Geometry: see drawing. Coordinates: mm, zero at the bounding-box minimum. A direction names the side the tool comes from. Round coordinates to 2 decimals unless told otherwise and drop trailing zeros. Loops run counter-clockwise (first coordinate to the right, second up) from the corner with the lowest first, then second, coordinate; pieces in that order, holes last. Notation, with made-up numbers: M -8.5,-13.75 L 0.5,-13.75 A31 cw 0.5,23.25 Z; hole C 45.5,54.25 d8. An arc over 180 degrees is marked long. Answer as a JSON object with one key per item and string values.
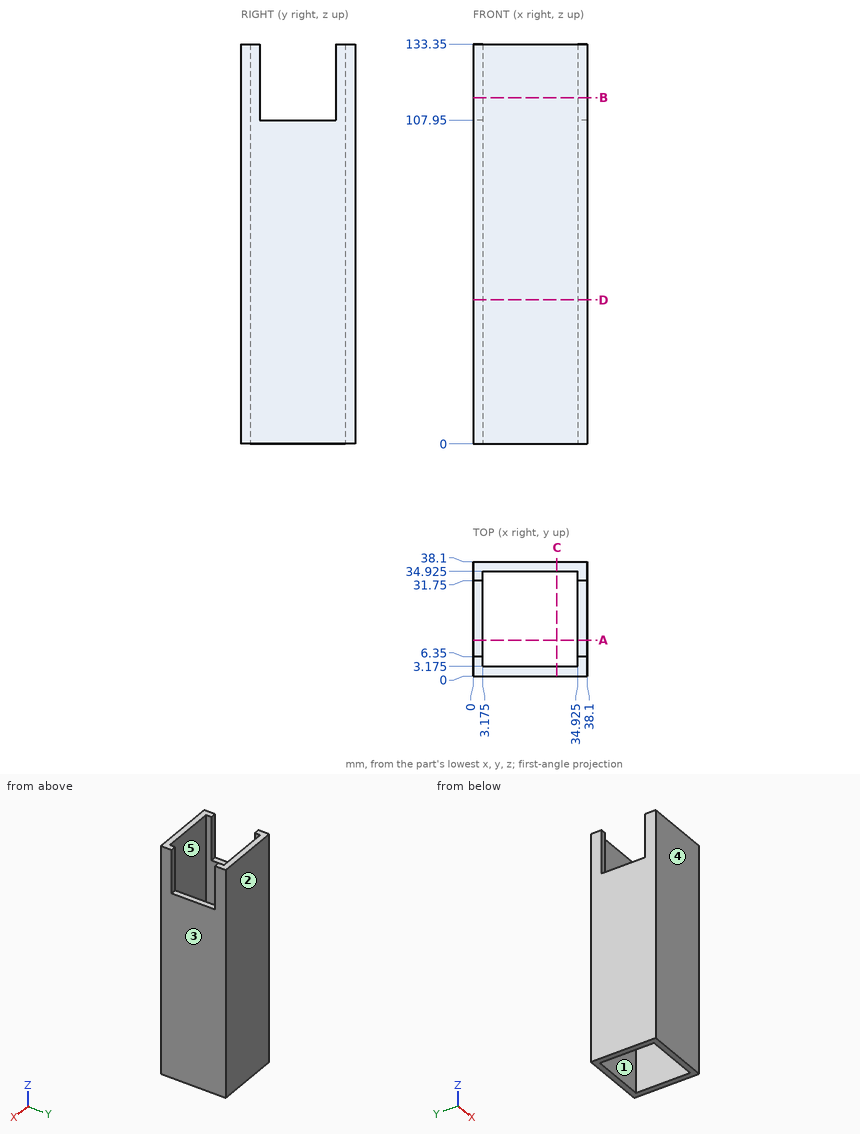
1) Pin query (flat end, axial travel): P1, Ø1.6, axis at x = 36.5, y = 14.5, coming from the +Z side. Return the tip coordinate at first contact, or that it passes through.
Results:
{"P1": "z = 107.95"}
2) Section query B-B (z = 115.5). Return the cut outline in (x, y) (3 decimals).
Results:
{"outline": "M 0,0 L 38.1,0 L 38.1,6.35 L 34.925,6.35 L 34.925,3.175 L 3.175,3.175 L 3.175,6.35 L 0,6.35 Z; M 0,31.75 L 3.175,31.75 L 3.175,34.925 L 34.925,34.925 L 34.925,31.75 L 38.1,31.75 L 38.1,38.1 L 0,38.1 Z"}
3) Ray query, line 1 (X direction, y = 8, z = 74) (3 decimals). Return the intervals inside material, ascending.
Results:
{"line 1": "0 to 3.175, 34.925 to 38.1"}
4) Reachability of the marked faces 1 and 2 from +Z, -Z, +X, -X, +Y, -Y: full face, straight path, thin tool, end or side. Return the list, or none.
Results:
{"face 1": "+Z, -Z", "face 2": "+Z, -Z, +X, -X, +Y"}
5) Section query C-C (x = 28). Return the cut outline in (y, z) (3 decimals), and give its area (3 significant figures).
Results:
{"outline": "M 0,0 L 3.175,0 L 3.175,133.35 L 0,133.35 Z; M 34.925,0 L 38.1,0 L 38.1,133.35 L 34.925,133.35 Z", "area": "847 mm2"}
6) Pull-direction query (X, two-part tool) for the marked faces 3, 4 and 5; classes: +X half, -X half, draft (parallel to the pull), parting line (faces both ways), or undercut.
Results:
{"face 3": "+X half", "face 4": "draft", "face 5": "undercut"}
7) Section query D-D (z = 48). Return the cut outline in (x, y) (3 decimals), and give its area (3 significant figures).
Results:
{"outline": "M 0,0 L 38.1,0 L 38.1,38.1 L 0,38.1 Z; hole M 3.175,3.175 L 34.925,3.175 L 34.925,34.925 L 3.175,34.925 Z", "area": "444 mm2"}
8) Section query A-A (y = 12). Return the cut outline in (x, z) (3 decimals), and give its area (3 significant figures).
Results:
{"outline": "M 0,0 L 3.175,0 L 3.175,107.95 L 0,107.95 Z; M 34.925,0 L 38.1,0 L 38.1,107.95 L 34.925,107.95 Z", "area": "685 mm2"}
